Verification items for the finished model (mm, model axes). A direction names the side the tool comes from. Coordinates: 2 decimals unless noted, no trailing zeros. Order: outer loops, then holes, each group sorted by start corner. A loop starts at its lowest first (then second) coordinate and runs counter-clockwise, first axis right, second up.
Q1. Cross-section at C-C, the plane y = -28.5. Record the boundary of the cut face in (x, z), and give its area (3 significant figures).
Q2. Draft check along Y on faces 1 (the flat face through (20, -44, -2)), 2 (the flat face through (10, -1, 10)), 3 (the flat face through (52, 49, -2)), 4 (the flat face through (-13, 57, 17)). Enter one of: pulls with the +Y half, pulls with the -Y half, needs draft (parallel to the pull), parting line crosses it, or undercut.
Q3. Cross-section at A-A, the plane x = -52.5. Record the boundary of the cut face in (y, z), and give its area (3 significant figures).
Q4. Set-up check for faces 5 (the flat face through (-51, -54, 0)), 6 (the flat face through (-15, -1, 7)), 7 (the flat face through (-53, 49, -2)), 8 (the flat face through (53, -49, -2)): record each of +Z, -Z, +X, -X, +Y, -Y from which the full face is reachable in a straight line by a thin tool's end or side.
Q5. Depth check by flat-ended pin: P1, Ø2.5, axis at x = 78.5, y = 54, coming from the -Z side; P2, Ø13.5, axis at x = -57, y = 49, coming from the +Z side; P3, Ø5, axis at y = 38, z = 15, coming from the -X side; P4, Ø3, axis at y = 10.5, z = 0, coming from the +X side. Enter the tip coordinate at first touch or a pass-through.
Q6. Cross-section at B-B, the plane z = 16.75. Record the boundary of the cut face in (x, y), and give its area (4 significant figures).
Q7. Thickness scan on line 1 (X direction, y = 50, z = 16.25); line 2 (Z direction, x = -12.45, y = -49); line 3 (Y direction, x = 73.5, z = -0.75). Record the ranges inside material, lowest first.
from build123d import *

# Parameters (mm, degrees)
SKETCH_R          = 1.5
PAD_DEPTH         = 5
SKETCH001_W       = 5
SKETCH001_H       = 118
PAD001_DEPTH      = 20
CHAMFER_SIZE      = 3
CHAMFER001_SIZE   = 5
CHAMFER002_SIZE   = 10
CHAMFER003_SIZE   = 3
SKETCH002_R       = 2.6
POCKET_DEPTH      = 17
POCKET_DEPTH_BACK = -100


with BuildPart() as part:
    # Sketch → Pad (new body)
    with BuildSketch(Plane.XY):
        Polygon((-83.5, 59), (-83.5, 49), (-15, 49), (-15, -49), (-83.5, -49), (-83.5, -59), (83.5, -59), (83.5, -49), (15, -49), (15, 49), (83.5, 49), (83.5, 59), align=None)
        with Locations((-78.5, 54)):
            Circle(SKETCH_R, mode=Mode.SUBTRACT)
        with Locations((78.5, 54)):
            Circle(SKETCH_R, mode=Mode.SUBTRACT)
        with Locations((78.5, -54)):
            Circle(SKETCH_R, mode=Mode.SUBTRACT)
        with Locations((-78.5, -54)):
            Circle(SKETCH_R, mode=Mode.SUBTRACT)
    extrude(amount=-PAD_DEPTH)

    # Sketch001 → Pad001 (join)
    with BuildSketch(Plane.XY):
        with Locations((-12.5, 0)):
            Rectangle(SKETCH001_W, SKETCH001_H)
        with Locations((12.5, 0)):
            Rectangle(SKETCH001_W, SKETCH001_H)
    extrude(amount=PAD001_DEPTH)

    # Chamfer
    chamfer_edges = [part.edges().sort_by_distance(p)[0] for p in [
        (-83.5, 49, -2.5),
        (-83.5, 59, -2.5),
        (-83.5, -49, -2.5),
        (-83.5, -59, -2.5),
        (83.5, -59, -2.5),
        (83.5, 49, -2.5),
        (83.5, 59, -2.5),
        (83.5, -49, -2.5),
    ]]
    chamfer(chamfer_edges, length=CHAMFER_SIZE)

    # Chamfer001
    chamfer001_edges = [part.edges().sort_by_distance(p)[0] for p in [
        (-12.5, -59, 20),
        (12.5, -59, 20),
        (12.5, 59, 20),
        (-12.5, 59, 20),
    ]]
    chamfer(chamfer001_edges, length=CHAMFER001_SIZE)

    # Chamfer002
    chamfer002_edges = [part.edges().sort_by_distance(p)[0] for p in [
        (-15, 49, -2.5),
        (-15, -49, -2.5),
        (15, -49, -2.5),
        (15, 49, -2.5),
    ]]
    chamfer(chamfer002_edges, length=CHAMFER002_SIZE)

    # Chamfer003
    chamfer003_edges = [part.edges().sort_by_distance(p)[0] for p in [
        (-15, 54, 0),
        (-15, -54, 0),
        (15, -54, 0),
        (15, 54, 0),
    ]]
    chamfer(chamfer003_edges, length=CHAMFER003_SIZE)

    # Sketch002 → Pocket (cut, two sides)
    with BuildSketch(Plane.YZ) as pocket_sk:
        with Locations((-49, 10)):
            Circle(SKETCH002_R)
        with Locations((49, 10)):
            Circle(SKETCH002_R)
    extrude(amount=-POCKET_DEPTH, mode=Mode.SUBTRACT)
    extrude(pocket_sk.sketch, amount=-POCKET_DEPTH_BACK, mode=Mode.SUBTRACT)


solid = part.part
Check values:
1. outline: (-15, -5) - (15, -5) - (15, 20) - (10, 20) - (10, 0) - (-10, 0) - (-10, 20) - (-15, 20) - close
1. area: 350 mm2
2. face 1: undercut
2. face 2: needs draft
2. face 3: undercut
2. face 4: pulls with the +Y half
3. outline: (-59, -5) - (-49, -5) - (-49, 0) - (-59, 0) - close; (49, -5) - (59, -5) - (59, 0) - (49, 0) - close
3. area: 100 mm2
4. face 5: +Z, -X, +Y, -Y
4. face 6: +Z, -X
4. face 7: +Z, -Z, -X
4. face 8: +Z, -Z, +X
5. P1: passes through
5. P2: stops at z = 0
5. P3: stops at x = -15
5. P4: stops at x = 15
6. outline: (-15, -57.25) - (-10, -57.25) - (-10, 57.25) - (-15, 57.25) - close; (10, -57.25) - (15, -57.25) - (15, 57.25) - (10, 57.25) - close
6. area: 1,145 mm2
7. line 1: x = -15 to -10, 10 to 15
7. line 2: z = -5 to 7.4, 12.6 to 20
7. line 3: y = -59 to -49, 49 to 59
